Here's how the part is built. I have some questions about the finished solid (model axes, mm). Face numbers are marked on the shaded views. A direction names the side the tool comes from. Round coordinates to 2 decimals unless told otherwise and drop trailing zeros. Write each loop counter-clockwise with the first axis right and the second up, starting at its lowest first coordinate (ties: lowest second). Pieces come first, ordered by that corner, then holes. Notation, with made-up numbers: (65, 77) - (108, 77) arc R20 ccw to (108, 100) - close; hole circle Ø5 at (-6, 67.5). An arc over 180 degrees is marked (long way). Use one line per item in the form item = value. Start each with the question number.
1. I want a section at D-D, the plane y = 1.25. List the corners of the cut face in (x, z) for me.
2. I want a section at B-B, the plane z = -13. List the corners of the cut face in (x, y) for me, plus the area to 3 significant figures.
3. We'd pull the mould along X, two halves only. Please class the marked faces 1, 2, 3 and 4: +X half, -X half, draft (parallel to the pull), parting line (faces both ways), or undercut.
4. I want a section at A-A, the plane y = 8.25. List the corners of the cut face in (x, z) for me, plus the area to 3 significant figures.
5. Will these pins go through, and if not, where does the flat tip stop? pin 1 (3.5 mm diameter, centred on x = -12, y = 7.5, fed in from +Z); pin 2 (1.5 mm diameter, centred on x = 22, z = 5, fed in from +Y); pin 3 (2 mm diameter, centred on y = 7.5, z = 7.5, fed in from +X); pin 4 (0.9 mm diameter, centred on y = 8, z = -2.5, fed in from -X).
6. If I drill on line 1 along Z through (x, y) = (16.5, 6.5); line 2 along Z through (x, y) = (-1, 5.5), over which ranges is the centre line in solid material (lowest first)?
7. Which directions (+Z, -Z, +X, -X, +Y, -Y) give clear straight access to the entire face, cutting with the end or side of a thin tool? Please do the marked faces 5 and 6.
8. I want a section at C-C, the plane x = 4.5. List the corners of the cut face in (y, z) for me, plus the area to 3 significant figures.
```python
from build123d import *

# Parameters (mm, degrees)
SKETCH1_W           = 56
SKETCH1_H           = 56
BOSS_EXTRUDE1_DEPTH = 2
SKETCH1_3_W         = 56
SKETCH1_3_H         = 56
SKETCH1_3_W_2       = 50
SKETCH1_3_H_2       = 50
BOSS_EXTRUDE2_DEPTH = 6
SKETCH2_W           = 52.7
SKETCH2_H           = 52.7
SKETCH2_W_2         = 50
SKETCH2_H_2         = 50
BOSS_EXTRUDE3_DEPTH = 3


with BuildPart() as part:
    # Sketch1 → Boss-Extrude1 (new body)
    with BuildSketch(Plane(origin=(0, 0, 0), x_dir=(1, 0, 0), z_dir=(0, 1, 0))):
        Rectangle(SKETCH1_W, SKETCH1_H)
    extrude(amount=-BOSS_EXTRUDE1_DEPTH)

    # Sketch1<3> → Boss-Extrude2 (add)
    with BuildSketch(Plane(origin=(0, 0, 0), x_dir=(1, 0, 0), z_dir=(0, 1, 0))):
        Rectangle(SKETCH1_3_W, SKETCH1_3_H)
        Rectangle(SKETCH1_3_W_2, SKETCH1_3_H_2, mode=Mode.SUBTRACT)
    extrude(amount=BOSS_EXTRUDE2_DEPTH)

    # Sketch2 → Boss-Extrude3 (add)
    with BuildSketch(Plane(origin=(0, 6, 0), x_dir=(1, 0, 0), z_dir=(0, 1, 0))):
        Rectangle(SKETCH2_W, SKETCH2_H)
        Rectangle(SKETCH2_W_2, SKETCH2_H_2, mode=Mode.SUBTRACT)
    extrude(amount=BOSS_EXTRUDE3_DEPTH)


solid = part.part
```
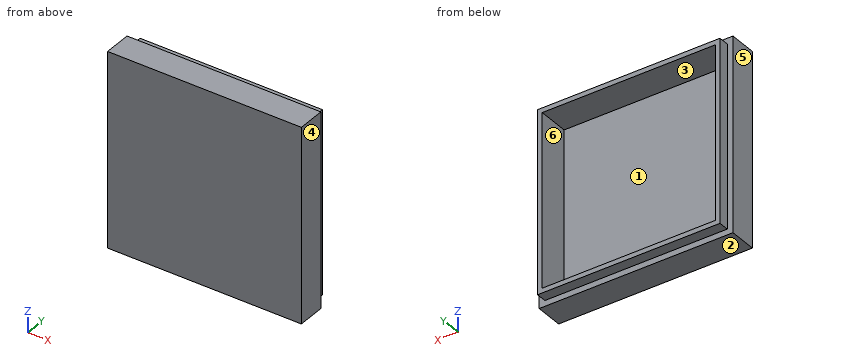
Model answer:
q1.outline = (-28, -28) - (28, -28) - (28, 28) - (-28, 28) - close; hole (-25, -25) - (25, -25) - (25, 25) - (-25, 25) - close
q2.outline = (-28, -2) - (28, -2) - (28, 6) - (26.35, 6) - (26.35, 9) - (25, 9) - (25, 0) - (-25, 0) - (-25, 9) - (-26.35, 9) - (-26.35, 6) - (-28, 6) - close
q2.area = 156 mm2
q3.face_1 = undercut
q3.face_2 = draft
q3.face_3 = undercut
q3.face_4 = +X half
q4.outline = (-26.35, -26.35) - (26.35, -26.35) - (26.35, 26.35) - (-26.35, 26.35) - close; hole (-25, -25) - (25, -25) - (25, 25) - (-25, 25) - close
q4.area = 277 mm2
q5.pin_1 = 28
q5.pin_2 = 0
q5.pin_3 = 26.35
q5.pin_4 = -26.35
q6.line_1 = -26.35 to -25, 25 to 26.35
q6.line_2 = -28 to -25, 25 to 28
q7.face_5 = +Z, -Z, -X, +Y, -Y
q7.face_6 = +Y
q8.outline = (-2, -28) - (6, -28) - (6, -26.35) - (9, -26.35) - (9, -25) - (0, -25) - (0, 25) - (9, 25) - (9, 26.35) - (6, 26.35) - (6, 28) - (-2, 28) - close
q8.area = 156 mm2
